Geometry: final body of the model. Coordinates: model frame, mm. A direction names the side the tool comes from. Give positions to 0.01 mm unless a question says otherwise; leave off trailing zeros. Loops run counter-clockwise (first coordinate to the right, second up) from the corner with the lowest first, then second, coordinate; pieces in that order, holes last. Notation, with made-up numbers: (-7.75, 10.5) -> (47.25, 10.5) arc R28 cw to (47.25, 32.5) -> close; hole circle Ø7 at (33, -25.75). An arc over 180 degrees is marked (long way). Answer in a Markdown table with one row per item. Add a question column.
1) Access query for faces 1 (the flat face through (-9.54, 4.47, -7.37)), 2 (the flat face through (-5, 2, -25.4)), 3 (the flat face through (-29.707, 4.472, 8.588)). Directions: +Z, -Z, +X, -X, +Y, -Y. A direction counts if a zero-diameter tool reaches every point of the face in a straight line with its end or side. Return the directions, or none.
2) First-contact query: P1, Ø5, axis at x = -22, z = -4, coming from the +Y side; P2, Ø3, axis at y = 5.5, z = -19, coming from the -X side; P3, Ø1.5, axis at x = -14.5, y = 2, coming from the -Z side. Flat tips, straight axial feed; report the tip coordinate or a pass-through.
3) Line query: line 1 (Y direction, x = -18.5, z = -3.5); line 2 (X direction, y = 3.5, z = -22.5); line 3 (Z direction, x = -19, y = 6.25). Output: solid intervals per line, ascending. Write a range as from..to.
4) Section query B-B (x = -23). Return the cut outline in (y, z), plus the area to 3 significant figures.
5) Section query C-C (z = -21). Return the cut outline in (x, y).
6) Section query A-A (y = 1.75). Return the cut outline in (x, z) (3 decimals).
```python
from build123d import *

# Parameters (mm, degrees)
BOSS_EXTRUDE1_DEPTH     = 6.35
FILLET1_R               = 9.525
CUT_EXTRUDE1_DEPTH      = 41.664797122
CUT_EXTRUDE1_DEPTH_BACK = 41.664797122
CUT_EXTRUDE2_DEPTH      = 3.81


with BuildPart() as part:
    # Sketch2 → Boss-Extrude1 (new body)
    with BuildSketch(Plane(origin=(0, 0, 0), x_dir=(1, 0, 0), z_dir=(0, 1, 0))):
        with BuildLine():
            Line((0, 0), (0, 25.4))
            Line((0, 25.4), (-12.7, 25.4))
            Line((-12.7, 25.4), (-30.807819057, -7.991432922))
            ThreePointArc((-30.807819057, -7.991432922), (-30.099929857, -11.233569232), (-26.7890625, -11.008375273))
            ThreePointArc((-26.7890625, -11.008375273), (-14.481351765, -2.859392016), (0, 0))
        make_face()
    extrude(amount=BOSS_EXTRUDE1_DEPTH)

    # Fillet1
    fillet1_edges = [part.edges().sort_by_distance(p)[0] for p in [
        (0, 3.175, 0),
    ]]
    fillet(fillet1_edges, radius=FILLET1_R)

    # Sketch3 → Cut-Extrude1 (cut, two sides: drawn at the far end of the back side and taken through both)
    with BuildSketch(Plane(origin=(0, 0, 0), x_dir=(-0.7071067811865489, 0, -0.7071067811865462), z_dir=(0.7071067811865462, 0, -0.7071067811865489)).offset(-CUT_EXTRUDE1_DEPTH_BACK)):
        with BuildLine():
            Line((9.525, 6.35), (9.525, 7.810784714))
            Line((9.525, 7.810784714), (2.20669647, 7.810784714))
            Line((2.20669647, 7.810784714), (2.20669647, 0))
            Line((2.20669647, 0), (3.175, 0))
            ThreePointArc((3.175, 0), (5.034871939, 4.490128061), (9.525, 6.35))
        make_face()
    extrude(amount=CUT_EXTRUDE1_DEPTH + CUT_EXTRUDE1_DEPTH_BACK, mode=Mode.SUBTRACT)

    # Sketch4 → Cut-Extrude2 (cut)
    with BuildSketch(Plane(origin=(0, 6.35, 0), x_dir=(1, 0, 0), z_dir=(0, 1, 0))):
        with BuildLine():
            Line((-16.337070041, 0.422049177), (-2.54, 14.52248663))
            Line((-2.54, 14.52248663), (-2.54, 25.4))
            Line((-2.54, 25.4), (-12.7, 25.4))
            Line((-12.7, 25.4), (-30.807819057, -7.991432922))
            Line((-30.807819057, -7.991432922), (-28.575, -9.202266957))
            ThreePointArc((-28.575, -9.202266957), (-22.702482164, -4.076735677), (-16.337070041, 0.422049177))
        make_face()
    extrude(amount=-CUT_EXTRUDE2_DEPTH, mode=Mode.SUBTRACT)


solid = part.part
```
Evaluation:
| question | item | result |
|---|---|---|
| 1 | face 1 | -Z, -X, +Y |
| 1 | face 2 | -Z, +X, -X, +Y, -Y |
| 1 | face 3 | -Z, +Y |
| 2 | P1 | y = 2.54 |
| 2 | P2 | x = -2.54 |
| 2 | P3 | z = -23.46 |
| 3 | line 1 | 0..2.54 |
| 3 | line 2 | -2.54..0 |
| 3 | line 3 | 1.34..5.08 |
| 4 | outline | (0, -6.41) -> (2.54, -6.41) -> (2.54, 4.31) -> (6.35, 4.31) -> (6.35, 7.73) -> (0, 7.73) -> close |
| 4 | area | 48.9 mm² |
| 5 | outline | (-15.09, 0) -> (0, 0) -> (0, 6.35) -> (-2.54, 6.35) -> (-2.54, 2.54) -> (-15.09, 2.54) -> close |
| 6 | outline | (-30.808, 7.991) -> (-12.7, -25.4) -> (0, -25.4) -> (0, -8.563) arc R9.525 ccw to (-1.686, -3.151) -> (-4.114, -0.724) arc R9.525 ccw to (-7.62, 0.77) arc R38.1 cw to (-26.789, 11.008) arc R2.54 ccw to start |
